from build123d import *

# Parameters (mm, degrees)
SKETCH1_W               = 425
SKETCH1_H               = 375
BOSS_EXTRUDE1_DEPTH     = 4.5
SKETCH2_R               = 7.5
CUT_EXTRUDE1_DEPTH      = 1
CUT_EXTRUDE1_DEPTH_BACK = 5.5


with BuildPart() as part:
    # Sketch1 → Boss-Extrude1 (new body)
    with BuildSketch(Plane.XY):
        Rectangle(SKETCH1_W, SKETCH1_H)
    extrude(amount=-BOSS_EXTRUDE1_DEPTH)

    # Sketch2 → Cut-Extrude1 (cut, two sides)
    with BuildSketch(Plane.XY) as cut_extrude1_sk:
        with Locations((-199.8, 87.5)):
            Circle(SKETCH2_R)
        with Locations((-100, 174.8)):
            Circle(SKETCH2_R)
        with Locations((100, 174.8)):
            Circle(SKETCH2_R)
        with Locations((199.8, 87.5)):
            Circle(SKETCH2_R)
        with Locations((-100, -174.8)):
            Circle(SKETCH2_R)
        with Locations((-199.8, -87.5)):
            Circle(SKETCH2_R)
        with Locations((199.8, -87.5)):
            Circle(SKETCH2_R)
        with Locations((100, -174.8)):
            Circle(SKETCH2_R)
    extrude(amount=CUT_EXTRUDE1_DEPTH, mode=Mode.SUBTRACT)
    extrude(cut_extrude1_sk.sketch, amount=-CUT_EXTRUDE1_DEPTH_BACK, mode=Mode.SUBTRACT)


solid = part.part
Geometry check sheet. Reference: the model listing, model coordinates, mm. Give positions to 0.01 mm unless a question says otherwise; leave off trailing zeros. Order: outer loops, then holes, each group sorted by start corner. A loop starts at its lowest first (then second) coordinate and runs counter-clockwise, first axis right, second up.
1. Sectioned sample at B-B (x = -199.8). Record the boundary of the cut face in (y, z), then the cut area to 3 significant figures.
Completed:
outline: (-187.5, -4.5) - (-95, -4.5) - (-95, 0) - (-187.5, 0) - close; (-80, -4.5) - (80, -4.5) - (80, 0) - (-80, 0) - close; (95, -4.5) - (187.5, -4.5) - (187.5, 0) - (95, 0) - close
area: 1,550 mm2
2. Draft check along Y on faces 1 (the face through (193.848, 82.936, -2.218)), 2 (the face through (-3, 3, -4.5)). Enter one of: pulls with the +Y half, pulls with the -Y half, needs draft (parallel to the pull), parting line crosses it, or undercut.
Completed:
face 1: undercut
face 2: needs draft
3. Depth check by flat-ended pin: pin 1 (9 mm diameter, centred on x = 100, y = -174.8, fed in from -Z). Enter the tip coordinate at first touch or a pass-through.
Completed:
pin 1: passes through
4. Scan lines: line 1 (Y direction, x = 199.8, z = -3.05); line 2 (Y direction, x = 100, z = -2.7). Record each from-to range of solid material in increasing order.
Completed:
line 1: y = -187.5 to -95, -80 to 80, 95 to 187.5
line 2: y = -187.5 to -182.3, -167.3 to 167.3, 182.3 to 187.5
5. Sectioned sample at A-A (y = -174.8). Record the boundary of the cut face in (x, z), then the cut area to 3 significant figures.
Completed:
outline: (-212.5, -4.5) - (-107.5, -4.5) - (-107.5, 0) - (-212.5, 0) - close; (-92.5, -4.5) - (92.5, -4.5) - (92.5, 0) - (-92.5, 0) - close; (107.5, -4.5) - (212.5, -4.5) - (212.5, 0) - (107.5, 0) - close
area: 1,780 mm2
